Model file for the job. Use its own axes, mm. Face numbers are marked on the shaded views. A direction names the side the tool comes from. Coordinates: 2 decimals unless noted, no trailing zeros. Loops run counter-clockwise (first coordinate to the right, second up) from the corner with the lowest first, then second, coordinate; pieces in that order, holes last. Notation, with made-up numbers: (39, 76.25) -> (54, 76.25) arc R21 ccw to (54, 97.25) -> close; hole circle Ø9 at (-28.75, -10). An arc over 180 degrees is marked (long way). Use one line per item in the form item = value.
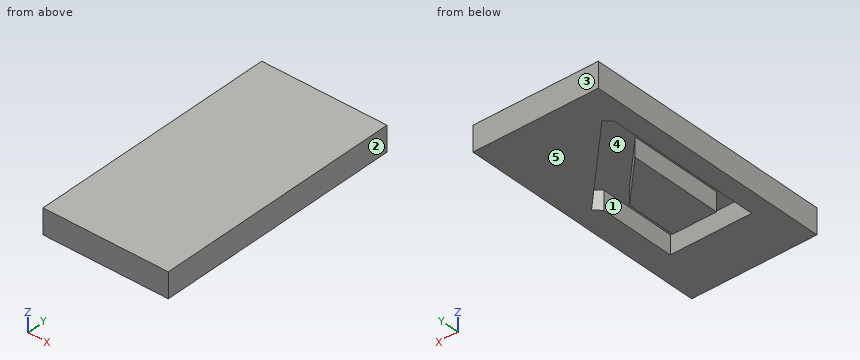
```python
from build123d import *

# Parameters (mm, degrees)
SKETCH1_W               = 40
SKETCH1_H               = 80
BOSS_EXTRUDE1_DEPTH     = 8
CUT_EXTRUDE_THIN1_DEPTH = 6
SKETCH2_W               = 6
SKETCH2_H               = 36.769552622
CUT_EXTRUDE1_DEPTH      = 3


with BuildPart() as part:
    # Sketch1 → Boss-Extrude1 (new body)
    with BuildSketch(Plane.XY):
        with Locations((-83.02277118, 5.318441745)):
            Rectangle(SKETCH1_W, SKETCH1_H)
    extrude(amount=BOSS_EXTRUDE1_DEPTH)

    # Sketch1<4> → Cut-Extrude-Thin1 (cut)
    with BuildSketch(Plane.XY):
        Polygon((-97.012604353, 32.561082432), (-97.012604353, -17.681558255), (-71.012604353, -17.681558255), (-71.012604353, 6.561082432), align=None)
        Polygon((-91.012604353, 18.075801058), (-91.012604353, -11.681558255), (-77.012604353, -11.681558255), (-77.012604353, 4.075801058), align=None, mode=Mode.SUBTRACT)
    extrude(amount=CUT_EXTRUDE_THIN1_DEPTH, mode=Mode.SUBTRACT)

    # Sketch2 → Cut-Extrude1 (cut)
    with BuildSketch(Plane(origin=(-32.22576096, -32.22576096, 0), x_dir=(0, 0, 1), z_dir=(-0.7071067811865461, -0.707106781186549, 0))):
        with Locations((3, 73.237656278)):
            Rectangle(SKETCH2_W, SKETCH2_H)
    extrude(amount=-CUT_EXTRUDE1_DEPTH, mode=Mode.SUBTRACT)


solid = part.part
```
Q1. Which spindle directions (+Z, -Z, +X, -X, +Y, -Y) get a long thin tool onto all of the face, cutting with end or side? Do the marked faces 1 and 2. Say none if no direction does.
Result:
face_1 = -Z
face_2 = +Z, -Z, +X, +Y, -Y
Q2. Band-saw the part on A-A, the plane z = 3. Write the cut outline in (x, y), and give its area (3 significant figures).
Result:
outline = (-103.02, -34.68) -> (-63.02, -34.68) -> (-63.02, 45.32) -> (-103.02, 45.32) -> close; (-91.01, -11.68) -> (-77.01, -11.68) -> (-77.01, 4.08) -> (-91.01, 18.08) -> close; hole (-97.01, -17.68) -> (-71.01, -17.68) -> (-71.01, 6.56) -> (-68.89, 8.68) -> (-94.89, 34.68) -> (-97.01, 32.56) -> close
area = 2,440 mm2
Q3. Band-saw the part on D-D, the plane y = 21. Write the cut outline in (x, z).
Result:
outline = (-103.02, 0) -> (-97.01, 0) -> (-97.01, 6) -> (-81.21, 6) -> (-81.21, 0) -> (-63.02, 0) -> (-63.02, 8) -> (-103.02, 8) -> close
Q4. Band-saw the part on B-B, the plane y = -3.5. Write the cut outline in (x, z).
Result:
outline = (-103.02, 0) -> (-97.01, 0) -> (-97.01, 6) -> (-91.01, 6) -> (-91.01, 0) -> (-77.01, 0) -> (-77.01, 6) -> (-71.01, 6) -> (-71.01, 0) -> (-63.02, 0) -> (-63.02, 8) -> (-103.02, 8) -> close
Q5. Band-saw the part on C-C, the plane x = -75.5. Write the cut outline in (y, z).
Result:
outline = (-34.68, 0) -> (-17.68, 0) -> (-17.68, 6) -> (15.29, 6) -> (15.29, 0) -> (45.32, 0) -> (45.32, 8) -> (-34.68, 8) -> close
Q6. Wall check: line 1 along X through (y, z) = (1, 4.5); line 2 along X through (y, z) = (-14, 3); line 3 along Y through (x, z) = (-83, 3.5). Give the ranges that are in metal, low to high.
Result:
line_1 = -103.02 to -97.01, -91.01 to -77.01, -71.01 to -63.02
line_2 = -103.02 to -97.01, -71.01 to -63.02
line_3 = -34.68 to -17.68, -11.68 to 10.06, 22.79 to 45.32
Q7. Mould opens along Y. For the marked faces 3, 4 and 5 say: released by +Y, released by -Y, zero draft, split by the parting line, or undercut.
Result:
face_3 = released by +Y
face_4 = undercut
face_5 = zero draft
